Can you work these out from the model? Positions are in its coordinate system, mm. A direction names the side the tool comes from. Coordinates: 2 decimals unless noted, no trailing zeros. Order: outer loops, then holes, each group sorted by start corner. A loop starts at its lowest first (then second) coordinate and runs counter-clockwise, first axis right, second up. Notation, with made-up numbers: M -6,78 L 22,78 A13 ccw 22,92 Z; hole C 60,46 d11. An arc over 180 degrees is marked long. Answer as CSV lines item,"result". Start each with the question number.
1. If we mould it in two halves opening along X, with no side actions, what happens to faces 1 (the face through (58, 1, 69)), 2 (the face through (31.54, 0.06, 100.15))? For each: released by +X, released by -X, zero draft, split by the parting line, or undercut.
2. Will these pins go through, and if not, where does the flat tip stop? pin 1 (13 mm diameter, centred on x = 86, z = -18.5, fed in from +Y); pin 2 (2 mm diameter, centred on y = -3, z = -52.5, fed in from -X); pin 3 (8 mm diameter, centred on x = 83, z = 46, fed in from -Y); pin 4 (21 mm diameter, centred on x = -6, z = -87, fed in from -Y).
3. I need wall thicknesses on line 1 along Z through (x, y) = (-62.5, 2); line 2 along X through (y, z) = (-1.5, 53.5); line 3 along X through (y, z) = (-3.3, 45). Which ranges of each line are inside material? Lowest first, please. Write a range as from..to.
4. If we section it at C-C (z = 65.5): List the corners of the cut face in (x, y) for me, plus the area to 3 significant figures.
5. On a 3-axis mill with a long thin cutter (end or side, diameter ignored), from which of +Z, -Z, +X, -X, +Y, -Y can I reach the whole of each face in a straight line? I mean faces 3 (the face through (58, -1, -69)), 4 (the face through (-70.542, 2.479, 66.126)). Say none if no direction works.
6. If we section it at B-B (z = 0): List the corners of the cut face in (x, y) for me.
7. If we section it at D-D (x = -49): List the corners of the cut face in (y, z) for me.
8. If we section it at A-A (x = 0): List the corners of the cut face in (y, z) for me.
```python
from build123d import *

# Parameters (mm, degrees)
SKETCH2_R           = 105
SKETCH2_R_2         = 7.5
SKETCH2_R_3         = 13
BOSS_EXTRUDE1_DEPTH = 4
SKETCH1_R           = 105
SKETCH1_R_2         = 7.5
BOSS_EXTRUDE2_DEPTH = 1


with BuildPart() as part:
    # Sketch2 → Boss-Extrude1 (new, symmetric)
    with BuildSketch(Plane(origin=(0, 0, 0), x_dir=(1, 0, 0), z_dir=(0, 1, 0))):
        with Locations(Location((0, 0, 0), (0, 0, 270))):
            Circle(SKETCH2_R)
        with Locations(Location((0, 0, 0), (0, 0, 270))):
            Circle(SKETCH2_R_2, mode=Mode.SUBTRACT)
        with Locations(Location((0, 90, 0), (0, 0, 270))):
            Circle(SKETCH2_R_3, mode=Mode.SUBTRACT)
        with Locations(Location((30.781812899, 84.572335871, 0), (0, 0, 270))):
            Circle(SKETCH2_R_3, mode=Mode.SUBTRACT)
        with Locations(Location((57.850884872, 68.943999881, 0), (0, 0, 270))):
            Circle(SKETCH2_R_3, mode=Mode.SUBTRACT)
        with Locations(Location((77.942286341, 45, 0), (0, 0, 270))):
            Circle(SKETCH2_R_3, mode=Mode.SUBTRACT)
        with Locations(Location((88.632697771, 15.62833599, 0), (0, 0, 270))):
            Circle(SKETCH2_R_3, mode=Mode.SUBTRACT)
        with Locations(Location((88.632697771, -15.62833599, 0), (0, 0, 270))):
            Circle(SKETCH2_R_3, mode=Mode.SUBTRACT)
        with Locations(Location((77.942286341, -45, 0), (0, 0, 270))):
            Circle(SKETCH2_R_3, mode=Mode.SUBTRACT)
        with Locations(Location((57.850884872, -68.943999881, 0), (0, 0, 270))):
            Circle(SKETCH2_R_3, mode=Mode.SUBTRACT)
        with Locations(Location((30.781812899, -84.572335871, 0), (0, 0, 270))):
            Circle(SKETCH2_R_3, mode=Mode.SUBTRACT)
        with Locations(Location((0, -90, 0), (0, 0, 270))):
            Circle(SKETCH2_R_3, mode=Mode.SUBTRACT)
        with Locations(Location((-30.781812899, -84.572335871, 0), (0, 0, 270))):
            Circle(SKETCH2_R_3, mode=Mode.SUBTRACT)
        with Locations(Location((-57.850884872, -68.943999881, 0), (0, 0, 270))):
            Circle(SKETCH2_R_3, mode=Mode.SUBTRACT)
        with Locations(Location((-77.942286341, -45, 0), (0, 0, 270))):
            Circle(SKETCH2_R_3, mode=Mode.SUBTRACT)
        with Locations(Location((-88.632697771, -15.62833599, 0), (0, 0, 270))):
            Circle(SKETCH2_R_3, mode=Mode.SUBTRACT)
        with Locations(Location((-88.632697771, 15.62833599, 0), (0, 0, 270))):
            Circle(SKETCH2_R_3, mode=Mode.SUBTRACT)
        with Locations(Location((-77.942286341, 45, 0), (0, 0, 270))):
            Circle(SKETCH2_R_3, mode=Mode.SUBTRACT)
        with Locations(Location((-57.850884872, 68.943999881, 0), (0, 0, 270))):
            Circle(SKETCH2_R_3, mode=Mode.SUBTRACT)
        with Locations(Location((-30.781812899, 84.572335871, 0), (0, 0, 270))):
            Circle(SKETCH2_R_3, mode=Mode.SUBTRACT)
    extrude(amount=BOSS_EXTRUDE1_DEPTH, both=True)

    # Sketch1 → Boss-Extrude2 (add, symmetric)
    with BuildSketch(Plane(origin=(0, 0, 0), x_dir=(1, 0, 0), z_dir=(0, 1, 0))):
        with Locations(Location((0, 0, 0), (0, 0, 270))):
            Circle(SKETCH1_R)
        with Locations(Location((0, 0, 0), (0, 0, 270))):
            Circle(SKETCH1_R_2, mode=Mode.SUBTRACT)
    extrude(amount=BOSS_EXTRUDE2_DEPTH, both=True)


solid = part.part
```
Solved:
1,face 1,"undercut"
1,face 2,"split by the parting line"
2,pin 1,"y = 1"
2,pin 2,"x = -91.5"
2,pin 3,"y = -1"
2,pin 4,"y = -4"
3,line 1,"-84.37..-81.08, -56.8..56.8, 81.08..84.37"
3,line 2,"-90.35..-87.78, -68.11..68.11, 87.78..90.35"
3,line 3,"-94.87..-90.94, -64.94..64.94, 90.94..94.87"
4,outline,"M -82.07,-4 L -70.39,-4 L -70.39,-1 L -45.32,-1 L -45.32,-4 L 45.32,-4 L 45.32,-1 L 70.39,-1 L 70.39,-4 L 82.07,-4 L 82.07,4 L 70.39,4 L 70.39,1 L 45.32,1 L 45.32,4 L -45.32,4 L -45.32,1 L -70.39,1 L -70.39,4 L -82.07,4 Z"
4,area,"1,010 mm²"
5,face 3,"-Y"
5,face 4,"+Y"
6,outline,"M -105,-4 L -7.5,-4 L -7.5,4 L -105,4 Z; M 7.5,-4 L 105,-4 L 105,4 L 7.5,4 Z"
7,outline,"M -4,-92.87 L 4,-92.87 L 4,-78.47 L 1,-78.47 L 1,-59.42 L 4,-59.42 L 4,59.42 L 1,59.42 L 1,78.47 L 4,78.47 L 4,92.87 L -4,92.87 L -4,78.47 L -1,78.47 L -1,59.42 L -4,59.42 L -4,-59.42 L -1,-59.42 L -1,-78.47 L -4,-78.47 Z"
8,outline,"M -4,-105 L 4,-105 L 4,-103 L 1,-103 L 1,-77 L 4,-77 L 4,-7.5 L -4,-7.5 L -4,-77 L -1,-77 L -1,-103 L -4,-103 Z; M -4,7.5 L 4,7.5 L 4,77 L 1,77 L 1,103 L 4,103 L 4,105 L -4,105 L -4,103 L -1,103 L -1,77 L -4,77 Z"
